```python
from build123d import *

# Parameters (mm, degrees)
SKETCH1_R           = 26.5
BOSS_EXTRUDE1_DEPTH = 19
SHELL1_T            = -4
SKETCH3_W           = 1.8
SKETCH3_H           = 3.2


with BuildPart() as part:
    # Sketch1 → Boss-Extrude1 (new, symmetric)
    with BuildSketch(Plane.XY):
        Circle(SKETCH1_R)
    extrude(amount=BOSS_EXTRUDE1_DEPTH, both=True)

    # Shell1
    shell1_openings = [part.faces().sort_by_distance(p)[0] for p in [
        (0, 0, 19),
    ]]
    offset(amount=SHELL1_T, openings=shell1_openings, kind=Kind.INTERSECTION)

    # Sketch3 → Cut-Revolve1 (revolve, cut)
    with BuildSketch(Plane(origin=(0, 0, 0), x_dir=(1, 0, 0), z_dir=(0, 1, 0))):
        with Locations((25.6, -10.2)):
            Rectangle(SKETCH3_W, SKETCH3_H)
    revolve(axis=Axis((0, 0, 19), (0, 0, -1)), mode=Mode.SUBTRACT)


solid = part.part
```
Could you check a few things on this model? Use its own coordinates, in mm. A direction names the side the tool comes from. Round coordinates to 2 decimals unless told otherwise and drop trailing zeros. Loops run counter-clockwise (first coordinate to the right, second up) from the corner with the lowest first, then second, coordinate; pieces in that order, holes last. Notation, with made-up numbers: M 42.5,59.5 L 97.5,59.5 A17 cw 97.5,90.5 Z; hole C 57,8 d3. An arc over 180 degrees is marked long. Answer as CSV lines item,"result".
1) We'd pull the mould along X, two halves only. Please class faces 1 (the cylindrical face through (10.382, -19.961, 2.238)), 2 (the cylindrical face through (14.246, 22.345, 15.45)), 3 (the flat face through (22, -12, 11.8)): released by +X, released by -X, zero draft, split by the parting line, or undercut.
From the geometry:
face 1,"undercut"
face 2,"split by the parting line"
face 3,"zero draft"
2) Imagine slicing it at A-A on x = 0. List the corners of the cut face in (y, z) for me.
From the geometry:
outline,"M -26.5,-19 L 26.5,-19 L 26.5,8.6 L 24.7,8.6 L 24.7,11.8 L 26.5,11.8 L 26.5,19 L 22.5,19 L 22.5,-15 L -22.5,-15 L -22.5,19 L -26.5,19 L -26.5,11.8 L -24.7,11.8 L -24.7,8.6 L -26.5,8.6 Z"
3) For pin 1 Ø1 at (y, z) = (-14.5, 15) entering from +X; pin 2 Ø13.5 at (x, y) = (5.5, 5) entering from +Z; pin 3 Ø12 at (y, z) = (4.5, -5) entering from -X; pin 4 Ø2 at (y, z) = (-7, 7) entering from +X, each with a flat end and sliding along its axis, tell me the tip position at first contact or that it passes through.
From the geometry:
pin 1,"x = 22.5"
pin 2,"z = -15"
pin 3,"x = -26.5"
pin 4,"x = 25.81"
4) Which directions (+Z, -Z, +X, -X, +Y, -Y) give clear straight access to the entire face, cutting with the end or side of a thin tool? Please do faces 4 (the flat face through (0, 0, -15)), 5 (the flat face through (0, 0, -19)), 6 (the cylindrical face through (23.56, -7.42, 10.18)).
From the geometry:
face 4,"+Z"
face 5,"-Z, +X, -X, +Y, -Y"
face 6,"none"
5) Imagine slicing it at B-B on z = 4. List the corners of the cut face in (x, y) for me.
From the geometry:
outline,"C 0,0 d53; hole C 0,0 d45"
6) If I drill on probe 1 along Y at (x, z) = (0, 1.5); probe 2 along X at (y, z) = (6.5, 6.5); probe 3 along Y at (x, z) = (8.5, 3), over which ranges is the centre line in solid material (lowest first)?
From the geometry:
probe 1,"-26.5 to -22.5, 22.5 to 26.5"
probe 2,"-25.69 to -21.54, 21.54 to 25.69"
probe 3,"-25.1 to -20.83, 20.83 to 25.1"
